```python
from build123d import *

# Parameters (mm, degrees)
SKETCH1_W           = 80
SKETCH1_H           = 45
BOSS_EXTRUDE1_DEPTH = 42
SKETCH3_W           = 22
SKETCH3_H           = 28
CUT_EXTRUDE2_DEPTH  = 46
SKETCH4_W           = 10
SKETCH4_H           = 17
CUT_EXTRUDE3_DEPTH  = 28
SKETCH7_R           = 12
CUT_EXTRUDE5_DEPTH  = 3.5
SKETCH11_R          = 1.35
CUT_EXTRUDE6_DEPTH  = 15
SKETCH12_R          = 5.75
CUT_EXTRUDE7_DEPTH  = 42.5
SKETCH13_R          = 7.5
CUT_EXTRUDE8_DEPTH  = 46
SKETCH14_W          = 12.099538741
SKETCH14_H          = 10
CUT_EXTRUDE9_DEPTH  = 46
SKETCH15_R          = 1.712332532
CUT_EXTRUDE10_DEPTH = 43
SKETCH16_R          = 1.85
CUT_EXTRUDE11_DEPTH = 8
FILLET2_R           = 5
SKETCH17_R          = 12.5
CUT_EXTRUDE12_DEPTH = 31


with BuildPart() as part:
    # Sketch1 → Boss-Extrude1 (new body)
    with BuildSketch(Plane.XY):
        with Locations((40, 22.5)):
            Rectangle(SKETCH1_W, SKETCH1_H)
    extrude(amount=BOSS_EXTRUDE1_DEPTH)

    # Sketch3 → Cut-Extrude2 (cut, through all)
    with BuildSketch(Plane(origin=(0, 45, 0), x_dir=(1, 0, 0), z_dir=(0, 1, 0))):
        with Locations((11, -14)):
            Rectangle(SKETCH3_W, SKETCH3_H)
    extrude(amount=-CUT_EXTRUDE2_DEPTH, mode=Mode.SUBTRACT)

    # Sketch4 → Cut-Extrude3 (cut)
    with BuildSketch(Plane.ZY):
        with Locations((35, 22.5)):
            Rectangle(SKETCH4_W, SKETCH4_H)
    extrude(amount=-CUT_EXTRUDE3_DEPTH, mode=Mode.SUBTRACT)

    # Sketch7 → Cut-Extrude5 (cut)
    with BuildSketch(Plane(origin=(0, 45, 0), x_dir=(1, 0, 0), z_dir=(0, 1, 0))):
        with Locations((36, -21)):
            Circle(SKETCH7_R)
    extrude(amount=-CUT_EXTRUDE5_DEPTH, mode=Mode.SUBTRACT)

    # Sketch11 → Cut-Extrude6 (cut)
    with BuildSketch(Plane(origin=(0, 41.5, 0), x_dir=(1, 0, 0), z_dir=(0, 1, 0))):
        with Locations((41.656854249, -15.343145751)):
            Circle(SKETCH11_R)
        with Locations((41.656854249, -26.656854249)):
            Circle(SKETCH11_R)
        with Locations((30.343145751, -26.656854249)):
            Circle(SKETCH11_R)
        with Locations((30.343145751, -15.343145751)):
            Circle(SKETCH11_R)
    extrude(amount=-CUT_EXTRUDE6_DEPTH, mode=Mode.SUBTRACT)

    # Sketch12 → Cut-Extrude7 (cut, through all)
    with BuildSketch(Plane(origin=(0, 41.5, 0), x_dir=(1, 0, 0), z_dir=(0, 1, 0))):
        with Locations((36, -21)):
            Circle(SKETCH12_R)
    extrude(amount=-CUT_EXTRUDE7_DEPTH, mode=Mode.SUBTRACT)

    # Sketch13 → Cut-Extrude8 (cut, through all)
    with BuildSketch(Plane(origin=(0, 45, 0), x_dir=(1, 0, 0), z_dir=(0, 1, 0))):
        with Locations((66, -21)):
            Circle(SKETCH13_R)
    extrude(amount=-CUT_EXTRUDE8_DEPTH, mode=Mode.SUBTRACT)

    # Sketch14 → Cut-Extrude9 (cut, through all)
    with BuildSketch(Plane(origin=(0, 45, 0), x_dir=(1, 0, 0), z_dir=(0, 1, 0))):
        with Locations((73.950230629, -21)):
            Rectangle(SKETCH14_W, SKETCH14_H)
    extrude(amount=-CUT_EXTRUDE9_DEPTH, mode=Mode.SUBTRACT)

    # Sketch15 → Cut-Extrude10 (cut, through all)
    with BuildSketch(Plane.XY.offset(42)):
        with Locations((12.5, 22.500000001)):
            Circle(SKETCH15_R)
    extrude(amount=-CUT_EXTRUDE10_DEPTH, mode=Mode.SUBTRACT)

    # Sketch16 → Cut-Extrude11 (cut)
    with BuildSketch(Plane.XY.offset(42)):
        with Locations((10, 37.5)):
            Circle(SKETCH16_R)
        with Locations((70, 37.5)):
            Circle(SKETCH16_R)
        with Locations((70, 7.5)):
            Circle(SKETCH16_R)
        with Locations((10, 7.5)):
            Circle(SKETCH16_R)
    extrude(amount=-CUT_EXTRUDE11_DEPTH, mode=Mode.SUBTRACT)

    # Fillet2
    fillet2_edges = [part.edges().sort_by_distance(p)[0] for p in [
        (22, 22.5, 0),
        (22, 22.5, 28),
        (80, 22.5, 0),
    ]]
    fillet(fillet2_edges, radius=FILLET2_R)

    # Sketch17 → Cut-Extrude12 (cut)
    with BuildSketch(Plane.XZ):
        with Locations((36, 21)):
            Circle(SKETCH17_R)
    extrude(amount=-CUT_EXTRUDE12_DEPTH, mode=Mode.SUBTRACT)


solid = part.part
```
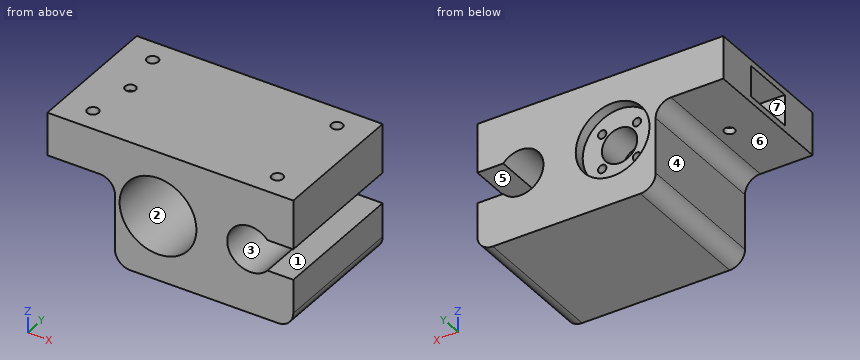
Input: part model. Units: mm. Frame: model coordinates. Face numbers are marked on the shaded views. A direction names the side the tool comes from. Round coordinates to 2 decimals unless told otherwise and drop trailing zeros. Loops run counter-clockwise (first coordinate to the right, second up) from the corner with the lowest first, then second, coordinate; pieces in that order, holes last. Notation, with made-up numbers: (13, 62.25) -> (55, 62.25) arc R24 cw to (55, 82.25) -> close; hole circle Ø10 at (85, 75). An arc over 180 degrees is marked (long way). Use one line per item in the form item = value. Start each with the question number.
Item 1: Section query C-C on x = 15.5. Return the cut outline in (y, z), then the cut area to 3 significant figures.
Item 2: Contact query for flat-ended pins moving along their axis: pin 1 Ø1.8 at (x, y) = (70, 8.5) entering from +Z; pin 2 Ø1.6 at (x, z) = (30.34, 26.66) entering from -Y; pin 3 Ø20 at (x, z) = (36, 21) entering from +Y; pin 4 Ø3 at (x, y) = (22.5, 36.5) entering from -Z. Output: stop coordinate, or through.
Item 3: Section query B-B on y = 11. Return the cut outline in (x, z).
Item 4: Material intervals for L1, parallel to Y at x = 10, z = 39.25; L2, parallel to X at y = 37, z = 36; L3, parallel to X at y = 36, z = 36.5, sorted ascending. Write a range as from..to.
Item 5: Section query A-A on x = 36. Return the cut outline in (y, z), then the cut area to 3 significant figures.
Item 6: Mould query, pull axis X, two halves, no side actions, for the marked faces 1, 2, 3 and 4. Classes: pulls with the +X half, pulls with the -X half, needs draft (parallel to the pull), parting line crosses it, or undercut.
Item 7: Section query D-D on y = 29. Return the cut outline in (x, z).
Item 8: Set-up query: the marked faces 5, 6 and 7. Return all of +Z, -Z, +X, -X, +Y, -Y with unobstructed straight access to the full face (end or side cutting, diameter ignored); none if empty.
Ans:
q1.outline = (0, 28) -> (45, 28) -> (45, 42) -> (0, 42) -> close; hole (14, 30) -> (31, 30) -> (31, 40) -> (14, 40) -> close
q1.area = 460 mm^2
q2.pin_1 = 42
q2.pin_2 = through
q2.pin_3 = 41.5
q2.pin_4 = 1
q3.outline = (0, 28) -> (17, 28) arc R5 cw to (22, 23) -> (22, 5) arc R5 ccw to (27, 0) -> (75, 0) arc R5 ccw to (80, 5) -> (80, 16) -> (71.59, 16) arc R7.5 cw (long way) to (71.59, 26) -> (80, 26) -> (80, 42) -> (0, 42) -> close; hole circle Ø25 at (36, 21)
q4.L1 = 0..5.65, 9.35..14, 31..35.65, 39.35..45
q4.L2 = 0..8.22, 11.78..68.22, 71.78..80
q4.L3 = 0..8.92, 11.08..68.92, 71.08..80
q5.outline = (0, 0) -> (45, 0) -> (45, 9) -> (41.5, 9) -> (41.5, 15.25) -> (31, 15.25) -> (31, 8.5) -> (0, 8.5) -> close; (0, 33.5) -> (31, 33.5) -> (31, 26.75) -> (41.5, 26.75) -> (41.5, 33) -> (45, 33) -> (45, 42) -> (0, 42) -> close
q5.area = 910 mm^2
q6.face_1 = needs draft
q6.face_2 = undercut
q6.face_3 = undercut
q6.face_4 = pulls with the -X half
q7.outline = (0, 28) -> (17, 28) arc R5 cw to (22, 23) -> (22, 5) arc R5 ccw to (27, 0) -> (75, 0) arc R5 ccw to (80, 5) -> (80, 16) -> (71.59, 16) arc R7.5 cw (long way) to (71.59, 26) -> (80, 26) -> (80, 42) -> (0, 42) -> (0, 40) -> (28, 40) -> (28, 30.6) arc R12.5 cw (long way) to (27.33, 30) -> (0, 30) -> close
q8.face_5 = +X, +Y, -Y
q8.face_6 = -Z, -X, +Y, -Y
q8.face_7 = -X
